```python
from build123d import *

# Parameters (mm, degrees)
IZIM2_R = 3


with BuildPart() as part:
    # Süpür1: sweep along a path in Çizim1
    with BuildLine(Plane.XY) as s_p_r1_path:
        Line((0, 0), (20, 0))
        ThreePointArc((20, 0), (27.071067812, 2.928932188), (30, 10))
        Line((30, 10), (30, 70))
        ThreePointArc((30, 70), (27.071067812, 77.071067812), (20, 80))
        Line((20, 80), (0, 80))
    # Çizim2 → Süpür1 (sweep)
    with BuildSketch(Plane(origin=(0, 0, 0), x_dir=(0, 0, -1), z_dir=(1, 0, 0))):
        Circle(IZIM2_R)
    sweep(path=s_p_r1_path.line)


solid = part.part
```
Part model, mm, in its own coordinate system. A direction names the side the tool comes from. Round coordinates to 2 decimals unless told otherwise and drop trailing zeros. Loops run counter-clockwise (first coordinate to the right, second up) from the corner with the lowest first, then second, coordinate; pieces in that order, holes last. Notation, with made-up numbers: (-25.5, 8) -> (5.5, 8) arc R19 ccw to (5.5, 35) -> close; hole circle Ø7 at (59.25, 49.25). An arc over 180 degrees is marked (long way). Use a Markdown table: item, result.
1) Pull direction Y, two halves, no side cores. Call faces 4 (the flat face through (0, 0, 0)), 5 (the cylindrical face through (10, 0, 3)): pulls with the +Y half, pulls with the -Y half, needs draft (parallel to the pull), parting line crosses it, or undercut.
The answers:
| item | result |
|---|---|
| face 4 | needs draft |
| face 5 | undercut |
2) Drop flat-ended pins along their axis: pin 1 Ø2 at (x, z) = (24.5, -0.5) entering from +Y; pin 2 Ø10 at (x, y) = (21.5, 8) entering from +Z; pin 3 Ø4 at (x, y) = (28, 60.5) entering from +Z. Give the stop position or say it passes through.
The answers:
| item | result |
|---|---|
| pin 1 | stops at y = 82.5 |
| pin 2 | stops at z = 1.66 |
| pin 3 | stops at z = 3 |
3) Cut at B-B, the plane y = 23. List the corners of the cut face in (x, z).
The answers:
| item | result |
|---|---|
| outline | circle Ø6 at (30, 0) |
4) Cut at C-C, the plane z = -0.5. List the corners of the cut face in (x, y), and give its area (3 significant figures).
The answers:
| item | result |
|---|---|
| outline | (0, -2.96) -> (20, -2.96) arc R12.96 ccw to (32.96, 10) -> (32.96, 70) arc R12.96 ccw to (20, 82.96) -> (0, 82.96) -> (0, 77.04) -> (20, 77.04) arc R7.04 cw to (27.04, 70) -> (27.04, 10) arc R7.04 cw to (20, 2.96) -> (0, 2.96) -> close |
| area | 777 mm2 |
5) Probe line 1 (Y direction, x = 10.5, z = 2.25); line 2 (Y direction, x = 7.5, z = 0.5); line 3 (X direction, y = 36, z = 0). List the from-to ranges inside material, lowest first. Write a range as [from, to].
The answers:
| item | result |
|---|---|
| line 1 | y = [-1.98, 1.98], [78.02, 81.98] |
| line 2 | y = [-2.96, 2.96], [77.04, 82.96] |
| line 3 | x = [27, 33] |
6) Tool access for faces 1 (the cylindrical face through (9.86, 82.93, 0.65)), 2 (the cylindrical face through (32.93, 40.42, 0.65)), 3 (the flat face through (0, 80, 0)): list every direction of +Z, -Z, +X, -X, +Y, -Y with a clear straight run to the whole face (end or side of a thin tool).
The answers:
| item | result |
|---|---|
| face 1 | -X |
| face 2 | none |
| face 3 | +Z, -Z, -X, +Y, -Y |
7) Cut at A-A, the plane x = 9.5. List the corners of the cut face in (y, z), and give its area (3 significant figures).
The answers:
| item | result |
|---|---|
| outline | circle Ø6 at (0, 0); circle Ø6 at (80, 0) |
| area | 56.5 mm2 |
